```python
from build123d import *

# Parameters (mm, degrees)
SKETCH_1_R          = 2.5
EXTRUDE_1_DEPTH     = 8
CUT_EXTRUDE_1_REACH = 39.599
SKETCH_3_R          = 2.5
SKETCH_4_R          = 1.7
EXTRUDE_2_DEPTH     = 4
FILLET_1_R          = 1.5


with BuildPart() as part:
    # 스케치1 → 보스-돌출1 (new body)
    with BuildSketch(Plane.XY):
        with BuildLine():
            Line((0, 5), (9, 5))
            Line((9, 5), (9, 8))
            Line((9, 8), (14, 8))
            Line((14, 8), (18.5, 3.5))
            Line((18.5, 3.5), (18.5, -1.5))
            Line((18.5, -1.5), (5.766282201, -8.851815399))
            Line((5.766282201, -8.851815399), (2.9854348, -31.5))
            Line((2.9854348, -31.5), (0.968172025, -33.193012598))
            ThreePointArc((0.968172025, -33.193012598), (0.755084879, -33.221081572), (0.63959988, -33.039815981))
            Line((0.63959988, -33.039815981), (0.63959988, -30.183726788))
            Line((0.63959988, -30.183726788), (-1.805734914, -27.269490262))
            Line((-1.805734914, -27.269490262), (-2.445573418, -12))
            Line((-2.445573418, -12), (-5, -4.696574134))
            Line((-5, -4.696574134), (-5, 0))
            ThreePointArc((-5, 0), (-3.535533906, 3.535533906), (0, 5))
        make_face()
        Circle(SKETCH_1_R, mode=Mode.SUBTRACT)
    extrude(amount=EXTRUDE_1_DEPTH)

    # 컷-돌출1: up to this plane
    cut_extrude_1_end = Plane(origin=(18.5, -1.5, 8), z_dir=(-0.5000000000000013, 0.8660254037844378, 0))
    # 스케치3 → 컷-돌출1 (cut, up to the surface)
    with BuildSketch(Plane(origin=(0, -1.5, 0), x_dir=(1, 0, 0), z_dir=(0, 1, 0)), mode=Mode.PRIVATE) as cut_extrude_1_sk1:
        with Locations(Location((15.349608759, -4, 0), (0, 0, 270))):
            Circle(SKETCH_3_R)
    cut_extrude_1_tool1 = split(extrude(cut_extrude_1_sk1.sketch, amount=-CUT_EXTRUDE_1_REACH, mode=Mode.PRIVATE), bisect_by=cut_extrude_1_end, keep=Keep.BOTH, mode=Mode.PRIVATE)
    add(cut_extrude_1_tool1.solids().sort_by_distance((15.349609, -1.5, 4))[0], mode=Mode.SUBTRACT)

    # 스케치4 → 보스-돌출2 (add)
    with BuildSketch(Plane.XZ.offset(1.5)):
        with Locations(Location((15.349608759, 4, 0), (0, 0, 90))):
            Circle(SKETCH_4_R)
    extrude(amount=EXTRUDE_2_DEPTH)

    # 필렛1
    fillet_1_edges = [part.edges().sort_by_distance(p)[0] for p in [
        (15.349608759, -5.5, 2.3),
    ]]
    fillet(fillet_1_edges, radius=FILLET_1_R)


solid = part.part
```
Read the model definition and answer for the solid it produces. Units are mm, in the model's axes. A direction names the side the tool comes from. Give positions to 0.01 mm unless a question says otherwise; leave off trailing zeros. Write each loop counter-clockwise with the first axis right and the second up, starting at its lowest first coordinate (ties: lowest second). Pieces come first, ordered by that corner, then holes. Notation, with made-up numbers: (27.25, 31) - (80.25, 31) arc R15 ccw to (80.25, 59) - close; hole circle Ø10 at (23, 88). An arc over 180 degrees is marked (long way). Write item = value, one per line. Start each with the question number.
Item 1: Find section B-B (x = 9.5). Give the vertices of the cut face in (y, z).
Item 2: The mould has two halves that part along X. Classify faces 5 (the cylindrical face through (16, -2.73, 5.57)), 6 (the flat face through (-3.705, -8.399, 3.944)), 7 (the flat face through (15, -1.5, 6)), 8 (the flat face through (16, 6, 4)): +X half, -X half, draft (parallel to the pull), parting line (faces both ways), or undercut.
Item 3: Find the intervals of material crossed by probe 1 along X at (y, z) = (-2, 1.75); probe 2 along X at (y, z) = (-2.9, 4); probe 3 along X at (y, z) = (-14.5, 2.75), in increasing order. Write a range as [from, to].
Item 4: Each of these flat-tipped pins is pushed along its axis until it touches: P1, Ø1.5, axis at x = 3, z = 2, coming from the -Y side; P2, Ø1, axis at x = 12, z = 5, coming from the -Y side; P3, Ø4, axis at x = 3.5, z = 2.5, coming from the +Y side. Where does it stop, or does it pass through?
Item 5: A tool of negligible diameter and unlimited length cuts with its end or side. For faces 1 (the flat face through (1.991, -32.335, 3.944)), 2 (the flat face through (4, 5, 4)), 3 (the cylindrical face through (12.9, -2.8, 3.5)), 4 (the flat face through (0.64, -32, 4)), from which of +Z, -Z, +X, -X, +Y, -Y can it reach the whole face along a straight path? Write none if from no direction.
Item 6: Find section A-A (y = 4). Give the vertices of the cut face in (x, z).
Response:
q1.outline = (-6.7, 0) - (8, 0) - (8, 8) - (-6.7, 8) - close
q2.face_5 = undercut
q2.face_6 = -X half
q2.face_7 = undercut
q2.face_8 = +X half
q3.probe_1 = [-5, -1.5], [1.5, 14.26], [16.44, 17.63]
q3.probe_2 = [-5, 12.85], [13.65, 17.05]
q3.probe_3 = [-2.34, 5.07]
q4.P1 = -32.12
q4.P2 = -5.54
q4.P3 = 5
q5.face_1 = +Z, -Z, +X, -Y
q5.face_2 = +Z, -Z, -X, +Y
q5.face_3 = -Y
q5.face_4 = +Z, -Z, -X, -Y
q6.outline = (-3, 0) - (18, 0) - (18, 8) - (-3, 8) - close
